from build123d import *

# Parameters (mm, degrees)
SKETCH1_R            = 3
SKETCH1_R_2          = 1.75
SKETCH1_R_3          = 1.5
BOSS_EXTRUDE2_DEPTH  = 3
SKETCH3_W            = 15.09800494
SKETCH3_H            = 15
CUT_EXTRUDE1_DEPTH   = 1.5
BOSS_EXTRUDE5_DEPTH  = 1.5
SKETCH5_W            = 5
SKETCH5_H            = 5
CUT_EXTRUDE2_DEPTH   = 1.5
BOSS_EXTRUDE7_DEPTH  = 3
SKETCH11_W           = 5
SKETCH11_H           = 5
BOSS_EXTRUDE11_DEPTH = 1.5
BOSS_EXTRUDE13_START = -3
SKETCH13_R           = 1.5
BOSS_EXTRUDE13_DEPTH = 3
SKETCH14_R           = 1.5
CUT_EXTRUDE6_DEPTH   = 103.094396255
SKETCH15_R           = 1.75
BOSS_EXTRUDE14_DEPTH = 3
SKETCH16_R           = 1.75
CUT_EXTRUDE7_DEPTH   = 103.094396255
SKETCH17_R           = 2.254560192
SKETCH17_R_2         = 2.966312922
SKETCH17_R_3         = 2.636452531
SKETCH17_R_4         = 1.99649084
SKETCH17_R_5         = 2.524996951
SKETCH17_R_6         = 3.313056584
SKETCH17_R_7         = 2.262213741
SKETCH17_R_8         = 2.353292134
BOSS_EXTRUDE15_DEPTH = 3
SKETCH19_R           = 1.75
CUT_EXTRUDE10_DEPTH  = 10
CUT_EXTRUDE11_DEPTH  = 10


with BuildPart() as part:
    # Sketch1 → Boss-Extrude2 (new body)
    with BuildSketch(Plane(origin=(0, 0, 0), x_dir=(1, 0, 0), z_dir=(0, 1, 0))):
        with BuildLine():
            Line((-7.45099753, -61.780902979), (-7.45099753, 61.780902979))
            ThreePointArc((-7.45099753, 61.780902979), (-8.239083338, 68.275631842), (-10.557599248, 74.393398282))
            ThreePointArc((-10.557599248, 74.393398282), (0.04900247, 100), (10.655604188, 74.393398282))
            ThreePointArc((10.655604188, 74.393398282), (8.337088278, 68.275631842), (7.54900247, 61.780902979))
            Line((7.54900247, 61.780902979), (7.54900247, -61.780902979))
            ThreePointArc((7.54900247, -61.780902979), (8.337088278, -68.275631842), (10.655604188, -74.393398282))
            ThreePointArc((10.655604188, -74.393398282), (0.04900247, -100), (-10.557599248, -74.393398282))
            ThreePointArc((-10.557599248, -74.393398282), (-8.239083338, -68.275631842), (-7.45099753, -61.780902979))
        make_face()
        with Locations(Location((0.04900247, 85, 0), (0, 0, 270))):
            Circle(SKETCH1_R, mode=Mode.SUBTRACT)
        with Locations(Location((-6.668511951, 91.717514421, 0), (0, 0, 270))):
            Circle(SKETCH1_R_2, mode=Mode.SUBTRACT)
        with Locations(Location((-5.607851779, 79.343145751, 0), (0, 0, 270))):
            Circle(SKETCH1_R_2, mode=Mode.SUBTRACT)
        with Locations(Location((5.70585672, 90.656854249, 0), (0, 0, 270))):
            Circle(SKETCH1_R_2, mode=Mode.SUBTRACT)
        with Locations(Location((6.766516891, 78.282485579, 0), (0, 0, 270))):
            Circle(SKETCH1_R_2, mode=Mode.SUBTRACT)
        with Locations(Location((0, 20, 0), (0, 0, 270))):
            Circle(SKETCH1_R_3, mode=Mode.SUBTRACT)
        with Locations(Location((5.70585672, -90.656854249, 0), (0, 0, 90))):
            Circle(SKETCH1_R_2, mode=Mode.SUBTRACT)
        with Locations(Location((-6.668511951, -91.717514421, 0), (0, 0, 90))):
            Circle(SKETCH1_R_2, mode=Mode.SUBTRACT)
        with Locations(Location((0.04900247, -85, 0), (0, 0, 90))):
            Circle(SKETCH1_R, mode=Mode.SUBTRACT)
        with Locations(Location((6.766516891, -78.282485579, 0), (0, 0, 90))):
            Circle(SKETCH1_R_2, mode=Mode.SUBTRACT)
        with Locations(Location((-5.607851779, -79.343145751, 0), (0, 0, 90))):
            Circle(SKETCH1_R_2, mode=Mode.SUBTRACT)
        with Locations(Location((0, -20, 0), (0, 0, 90))):
            Circle(SKETCH1_R_3, mode=Mode.SUBTRACT)
    extrude(amount=BOSS_EXTRUDE2_DEPTH)

    # Sketch3 → Cut-Extrude1 (cut)
    with BuildSketch(Plane(origin=(0, 3, 0), x_dir=(1, 0, 0), z_dir=(0, 1, 0))):
        Rectangle(SKETCH3_W, SKETCH3_H)
    extrude(amount=-CUT_EXTRUDE1_DEPTH, mode=Mode.SUBTRACT)

    # Sketch4 → Boss-Extrude5 (add, symmetric)
    with BuildSketch(Plane(origin=(0, 1.5, 0), x_dir=(1, 0, 0), z_dir=(0, 1, 0))):
        Polygon((7.54900247, -7.5), (19.98054828, -7.5), (7.54900247, -19.723921291), align=None)
        Polygon((-7.208608823, 7.5), (-20.353519271, 7.5), (-7.208608823, 20.276078709), align=None)
    extrude(amount=BOSS_EXTRUDE5_DEPTH, both=True)

    # Sketch5 → Cut-Extrude2 (cut)
    with BuildSketch(Plane(origin=(0, 3, 0), x_dir=(1, 0, 0), z_dir=(0, 1, 0))):
        with Locations((5.04900247, 10)):
            Rectangle(SKETCH5_W, SKETCH5_H)
        with Locations((-4.95099753, -10)):
            Rectangle(SKETCH5_W, SKETCH5_H)
    extrude(amount=-CUT_EXTRUDE2_DEPTH, mode=Mode.SUBTRACT)

    # Sketch6 → Boss-Extrude7 (add)
    with BuildSketch(Plane(origin=(0, 3, 0), x_dir=(1, 0, 0), z_dir=(0, 1, 0))):
        with BuildLine():
            Line((7.54900247, -19.723921291), (8.975074609, -18.321666587))
            ThreePointArc((8.975074609, -18.321666587), (7.919938782, -19.879401108), (7.54900247, -21.723921291))
            Line((7.54900247, -21.723921291), (7.54900247, -19.723921291))
        make_face()
        with BuildLine():
            Line((-7.45099753, 20.040491163), (-8.885188865, 18.646541661))
            ThreePointArc((-8.885188865, 18.646541661), (-7.824264446, 20.198223674), (-7.45099753, 22.040491163))
            Line((-7.45099753, 22.040491163), (-7.45099753, 20.040491163))
        make_face()
    extrude(amount=-BOSS_EXTRUDE7_DEPTH)

    # Sketch11 → Boss-Extrude11 (add)
    with BuildSketch(Plane(origin=(0, 1.5, 0), x_dir=(1, 0, 0), z_dir=(0, 1, 0))):
        with Locations((10.04900247, -5)):
            Rectangle(SKETCH11_W, SKETCH11_H)
        with Locations((-9.95099753, 5)):
            Rectangle(SKETCH11_W, SKETCH11_H)
    extrude(amount=-BOSS_EXTRUDE11_DEPTH)

    # Sketch13 → Boss-Extrude13 (add)
    with BuildSketch(Plane(origin=(0, 3, 0), x_dir=(1, 0, 0), z_dir=(0, 1, 0)).offset(BOSS_EXTRUDE13_START)):
        with Locations((0, -20)):
            Circle(SKETCH13_R)
        with Locations((0, 20)):
            Circle(SKETCH13_R)
    extrude(amount=BOSS_EXTRUDE13_DEPTH)

    # Sketch14 → Cut-Extrude6 (cut, through all)
    with BuildSketch(Plane(origin=(0, 3, 0), x_dir=(1, 0, 0), z_dir=(0, 1, 0))):
        with Locations(Location((-0.220863586, -21.21320344, 0), (0, 0, 270))):
            Circle(SKETCH14_R)
        with Locations(Location((-0.220863586, 21.2132, 0), (0, 0, 270))):
            Circle(SKETCH14_R)
    extrude(amount=-CUT_EXTRUDE6_DEPTH, mode=Mode.SUBTRACT)

    # Sketch15 → Boss-Extrude14 (add, through all)
    with BuildSketch(Plane(origin=(0, 3, 0), x_dir=(1, 0, 0), z_dir=(0, 1, 0))):
        with Locations((-5.607851779, 79.343145751)):
            Circle(SKETCH15_R)
        with Locations((6.766516891, 78.282485579)):
            Circle(SKETCH15_R)
        with Locations((-6.668511951, 91.717514421)):
            Circle(SKETCH15_R)
        with Locations((5.70585672, 90.656854249)):
            Circle(SKETCH15_R)
    extrude(amount=-BOSS_EXTRUDE14_DEPTH)

    # Sketch16 → Cut-Extrude7 (cut, through all)
    with BuildSketch(Plane(origin=(0, 3, 0), x_dir=(1, 0, 0), z_dir=(0, 1, 0))):
        with Locations(Location((-6.668511951, 78.282485579, 0), (0, 0, 270))):
            Circle(SKETCH16_R)
        with Locations(Location((5.70585672, 79.343145751, 0), (0, 0, 270))):
            Circle(SKETCH16_R)
        with Locations(Location((6.766516891, 91.717514421, 0), (0, 0, 270))):
            Circle(SKETCH16_R)
        with Locations(Location((-5.610118231, 90.659120701, 0), (0, 0, 270))):
            Circle(SKETCH16_R)
    extrude(amount=-CUT_EXTRUDE7_DEPTH, mode=Mode.SUBTRACT)

    # Sketch17 → Boss-Extrude15 (add)
    with BuildSketch(Plane(origin=(0, 3, 0), x_dir=(1, 0, 0), z_dir=(0, 1, 0))):
        with Locations((5.70585672, 79.343145751)):
            Circle(SKETCH17_R)
        with Locations((-6.668511951, 78.282485579)):
            Circle(SKETCH17_R_2)
        with Locations((-5.610118231, 90.659120701)):
            Circle(SKETCH17_R_3)
        with Locations((6.766516891, 91.717514421)):
            Circle(SKETCH17_R_4)
        with Locations((-6.668511951, -91.717514421)):
            Circle(SKETCH17_R_5)
        with Locations((-5.607851779, -79.343145751)):
            Circle(SKETCH17_R_6)
        with Locations((6.766516891, -78.282485579)):
            Circle(SKETCH17_R_7)
        with Locations((5.70585672, -90.656854249)):
            Circle(SKETCH17_R_8)
    extrude(amount=-BOSS_EXTRUDE15_DEPTH)

    # Sketch19 → Cut-Extrude10 (cut)
    with BuildSketch(Plane(origin=(0, 3, 0), x_dir=(1, 0, 0), z_dir=(0, 1, 0))):
        with Locations(Location((-0.220863586, -21.21320344, 0), (0, 0, 270))):
            Circle(SKETCH19_R)
        with Locations(Location((-0.220863586, 21.2132, 0), (0, 0, 270))):
            Circle(SKETCH19_R)
    extrude(amount=-CUT_EXTRUDE10_DEPTH, mode=Mode.SUBTRACT)

    # Sketch18 → Cut-Extrude11 (cut)
    with BuildSketch(Plane(origin=(0, 3, 0), x_dir=(1, 0, 0), z_dir=(0, 1, 0))):
        with BuildLine():
            Line((8.893452608, -93.844450138), (2.877429595, -87.828427125))
            ThreePointArc((2.877429595, -87.828427125), (2.364866462, -89.065863992), (2.877429595, -90.303300859))
            Line((2.877429595, -90.303300859), (6.418578874, -93.844450138))
            ThreePointArc((6.418578874, -93.844450138), (7.656015741, -94.357013271), (8.893452608, -93.844450138))
        make_face()
        with BuildLine():
            ThreePointArc((5.352303329, -87.828427125), (4.114866462, -87.315863992), (2.877429595, -87.828427125))
            Line((2.877429595, -87.828427125), (8.893452608, -93.844450138))
            ThreePointArc((8.893452608, -93.844450138), (9.406015741, -92.607013271), (8.893452608, -91.369576404))
            Line((8.893452608, -91.369576404), (5.352303329, -87.828427125))
        make_face()
        with BuildLine():
            Line((8.893452608, -76.155549862), (2.877429595, -82.171572875))
            ThreePointArc((2.877429595, -82.171572875), (4.114866462, -82.684136008), (5.352303329, -82.171572875))
            Line((5.352303329, -82.171572875), (8.893452608, -78.630423596))
            ThreePointArc((8.893452608, -78.630423596), (9.406015741, -77.392986729), (8.893452608, -76.155549862))
        make_face()
        with BuildLine():
            ThreePointArc((2.877429595, -79.696699141), (2.364866462, -80.934136008), (2.877429595, -82.171572875))
            Line((2.877429595, -82.171572875), (8.893452608, -76.155549862))
            ThreePointArc((8.893452608, -76.155549862), (7.656015741, -75.642986729), (6.418578874, -76.155549862))
            Line((6.418578874, -76.155549862), (2.877429595, -79.696699141))
        make_face()
        with BuildLine():
            Line((-8.795447668, -91.369576404), (-5.254298389, -87.828427125))
            ThreePointArc((-5.254298389, -87.828427125), (-2.779424655, -87.828427125), (-2.779424655, -90.303300859))
            Line((-2.779424655, -90.303300859), (-6.320573934, -93.844450138))
            ThreePointArc((-6.320573934, -93.844450138), (-8.795447668, -93.844450138), (-8.795447668, -91.369576404))
        make_face()
        with BuildLine():
            ThreePointArc((-5.254298389, -82.171572875), (-4.016861522, -82.684136008), (-2.779424655, -82.171572875))
            Line((-2.779424655, -82.171572875), (-8.795447668, -76.155549862))
            ThreePointArc((-8.795447668, -76.155549862), (-9.308010801, -77.392986729), (-8.795447668, -78.630423596))
            Line((-8.795447668, -78.630423596), (-5.254298389, -82.171572875))
        make_face()
        with BuildLine():
            Line((-8.795447668, -76.155549862), (-2.779424655, -82.171572875))
            ThreePointArc((-2.779424655, -82.171572875), (-2.266861522, -80.934136008), (-2.779424655, -79.696699141))
            Line((-2.779424655, -79.696699141), (-6.320573934, -76.155549862))
            ThreePointArc((-6.320573934, -76.155549862), (-7.558010801, -75.642986729), (-8.795447668, -76.155549862))
        make_face()
        with BuildLine():
            ThreePointArc((-2.779424655, 90.303300859), (-2.779424655, 87.828427125), (-5.254298389, 87.828427125))
            Line((-5.254298389, 87.828427125), (-8.795447668, 91.369576404))
            ThreePointArc((-8.795447668, 91.369576404), (-8.795447668, 93.844450138), (-6.320573934, 93.844450138))
            Line((-6.320573934, 93.844450138), (-2.779424655, 90.303300859))
        make_face()
        with BuildLine():
            Line((8.893452608, 91.369576404), (5.352303329, 87.828427125))
            ThreePointArc((5.352303329, 87.828427125), (2.877429595, 87.828427125), (2.877429595, 90.303300859))
            Line((2.877429595, 90.303300859), (6.418578874, 93.844450138))
            ThreePointArc((6.418578874, 93.844450138), (8.893452608, 93.844450138), (8.893452608, 91.369576404))
        make_face()
        with BuildLine():
            ThreePointArc((2.877429595, 79.696699141), (2.877429595, 82.171572875), (5.352303329, 82.171572875))
            Line((5.352303329, 82.171572875), (8.893452608, 78.630423596))
            ThreePointArc((8.893452608, 78.630423596), (8.893452608, 76.155549862), (6.418578874, 76.155549862))
            Line((6.418578874, 76.155549862), (2.877429595, 79.696699141))
        make_face()
        with BuildLine():
            Line((-8.795447668, 78.630423596), (-5.254298389, 82.171572875))
            ThreePointArc((-5.254298389, 82.171572875), (-2.779424655, 82.171572875), (-2.779424655, 79.696699141))
            Line((-2.779424655, 79.696699141), (-6.320573934, 76.155549862))
            ThreePointArc((-6.320573934, 76.155549862), (-8.795447668, 76.155549862), (-8.795447668, 78.630423596))
        make_face()
    extrude(amount=-CUT_EXTRUDE11_DEPTH, mode=Mode.SUBTRACT)


solid = part.part
Read the model definition and answer for the solid it produces. Units are mm, in the model's axes. A direction names the side the tool comes from. Coordinates: 2 decimals unless noted, no trailing zeros. Loops run counter-clockwise (first coordinate to the right, second up) from the corner with the lowest first, then second, coordinate; pieces in that order, holes last. Notation, with made-up numbers: (39, 47.25) - (69, 47.25) arc R19 ccw to (69, 75.25) - close; hole circle Ø4 at (77, 59.5). An arc over 180 degrees is marked (long way). Answer in a Markdown table with one row per item.
Q1. Given P1, Ø5.5, axis at x = 0.05, z = -85, coming from the +Y side; P2, Ø1.6, axis at x = -5, y = 2, coming from the -Z side; P3, Ø0.8, axis at y = 2.5, z = 9, coming from the -X side; P4, Ø1.6, axis at y = 1, z = -6, coming from the -X side, each flat-ended and moving along its own axis, determine where each tip first touches the part or whether it passes through.
Here are the results:
| item | result |
|---|---|
| P1 | passes through |
| P2 | stops at z = -99.39 |
| P3 | stops at x = -2.45 |
| P4 | stops at x = -12.45 |
Q2. Straight lines are drawn through the part: line 1 along X through (y, z) = (1.5, -85); line 2 along Z through (x, y) = (-0.5, 2.65); line 3 along Z through (x, y) = (-4, 2.7). For each, find the intervals that lie inside material, in ascending order. Write a range as [from, to].
Here are the results:
| item | result |
|---|---|
| line 1 | x = [-14.95, -2.95], [3.05, 15.05] |
| line 2 | z = [-99.99, -87.95], [-82.05, -22.94], [-19.49, -7.5], [7.5, 19.49], [22.94, 82.05], [87.95, 99.99] |
| line 3 | z = [-99.44, -91.52], [-87.32, -82.68], [-78.48, -7.5], [12.5, 78.48], [82.68, 87.32], [91.52, 99.44] |
Q3. Find section A-A on z = -85. Write down the section's boundary in (x, y), plus the area to 3 significant figures.
Here are the results:
| item | result |
|---|---|
| outline | (-14.95, 0) - (-2.95, 0) - (-2.95, 3) - (-14.95, 3) - close; (3.05, 0) - (15.05, 0) - (15.05, 3) - (3.05, 3) - close |
| area | 72.0 mm^2 |
Q4. For faces 4 (the flat face through (14.55, 1.48, 12.84)), 5 (the flat face through (3, 3, 53)), 6 (the flat face through (4.673, 1.521, -77.901)), 7 (the flat face through (-14.7, 1.521, -12.995)), determine the directions among +Z, -Z, +X, -X, +Y, -Y from which every point of the face is accessible in a straight line to the end or side of a thin tool.
Here are the results:
| item | result |
|---|---|
| face 4 | +X, +Y, -Y |
| face 5 | +Z, -Z, +X, -X, +Y |
| face 6 | +Y, -Y |
| face 7 | -X, +Y, -Y |
Q5. Find section B-B on y = 2. Count the separate pieces of the cut face and the enclosed holes in it, plus the area to 3 significant figures.
Here are the results:
| item | result |
|---|---|
| separate pieces | 2 |
| enclosed holes | 12 |
| area | 3,160 mm^2 |
Q6. Find section D-D on z = 68. Write down the section's boundary in (x, y), plus the area to 3 significant figures.
Here are the results:
| item | result |
|---|---|
| outline | (-8.17, 0) - (8.27, 0) - (8.27, 3) - (-8.17, 3) - close |
| area | 49.3 mm^2 |
Q7. Find section C-C on z = 29.5. Write down the section's boundary in (x, y).
Here are the results:
| item | result |
|---|---|
| outline | (-7.45, 0) - (7.55, 0) - (7.55, 3) - (-7.45, 3) - close |
Q8. The mould has two halves that part along X. Classify faces 1 (the flat face through (-7, 1.521, -89.574)), 2 (the cylindrical face through (8.36, 1.48, -68.36)), 3 (the flat face through (1, 3, -54)): pulls with the +X half, pulls with the -X half, needs draft (parallel to the pull), parting line crosses it, or undercut.
Here are the results:
| item | result |
|---|---|
| face 1 | undercut |
| face 2 | pulls with the +X half |
| face 3 | needs draft |
